```python
from build123d import *

# Parameters (mm, degrees)
SKETCH1_W           = 25.4
SKETCH1_H           = 25.4
BOSS_EXTRUDE1_DEPTH = 482.6
SKETCH2_R           = 6.35
BOSS_EXTRUDE2_DEPTH = 6.35
SKETCH3_R           = 6.35
BOSS_EXTRUDE3_DEPTH = 6.35
SKETCH4_W           = 25.4
SKETCH4_H           = 482.6
BOSS_EXTRUDE4_DEPTH = 18.288


with BuildPart() as part:
    # Sketch1 → Boss-Extrude1 (new body)
    with BuildSketch(Plane(origin=(0, 0, 0), x_dir=(1, 0, 0), z_dir=(0, 1, 0))):
        with Locations((12.7, 12.7)):
            Rectangle(SKETCH1_W, SKETCH1_H)
    extrude(amount=BOSS_EXTRUDE1_DEPTH)

    # Sketch2 → Boss-Extrude2 (add)
    with BuildSketch(Plane(origin=(25.4, 0, 0), x_dir=(0, 0, -1), z_dir=(1, 0, 0))):
        with Locations(Location((12.7, 469.9, 0), (0, 0, 180))):
            Circle(SKETCH2_R)
    extrude(amount=BOSS_EXTRUDE2_DEPTH)

    # Sketch3 → Boss-Extrude3 (add)
    with BuildSketch(Plane(origin=(25.4, 0, 0), x_dir=(0, 0, -1), z_dir=(1, 0, 0))):
        with Locations(Location((12.7, 12.7, 0), (0, 0, 180))):
            Circle(SKETCH3_R)
    extrude(amount=BOSS_EXTRUDE3_DEPTH)

    # Sketch4 → Boss-Extrude4 (add)
    with BuildSketch(Plane(origin=(0, 0, -25.4), x_dir=(-1, 0, 0), z_dir=(0, 0, -1))):
        with Locations((-12.7, 241.3)):
            Rectangle(SKETCH4_W, SKETCH4_H)
    extrude(amount=BOSS_EXTRUDE4_DEPTH)


solid = part.part
```
Check sheet for the modelled part. Datum: model origin and axes. Units: mm. Give positions to 0.01 mm unless a question says otherwise; leave off trailing zeros. Write each loop counter-clockwise with the first axis right and the second up, starting at its lowest first coordinate (ties: lowest second). Pieces come first, ordered by that corner, then holes. Notation, with made-up numbers: (81, 40) - (121, 40) arc R24 cw to (121, 76) - close; hole circle Ø1 at (63.5, -38). An arc over 180 degrees is marked (long way). Answer as a JSON object with one key per item and string values. Group by question number.
1) Depth check by flat-ended pin: P1, Ø8, axis at y = 247, z = -17, coming from the +X side; P2, Ø1.5, axis at x = 15.5, z = -35.5, coming from the -Y side. Enter the tip coordinate at first touch or a pass-through.
2) Sectioned sample at B-B (y = 12.7). Record the cut outline in (x, z), then the cut area to 3 significant figures.
3) Release check for a two-part mould opening along Y. For faces 1 (the face through (13, 0, -22)), 2 (the face through (13, 245, -43.688)), 3 (the face through (28.5, 463.6, -13.5)), 4 (the face through (28.53, 18.9, -14.08)) record: pulls with the +Y half, pulls with the -Y half, needs draft (parallel to the pull), parting line crosses it, or undercut.
4) Thickness scan on probe 1 along Y at (x, z) = (27.5, -13); probe 2 along X at (y, z) = (85, -36.5); probe 3 along Y at (x, z) = (30, -17.5). Record the ranges inside material, lowest first. Write a range as from..to.
5) Sectioned sample at C-C (z = -37). Record the cut outline in (x, y).
6) Sectioned sample at A-A (z = -12.7). Record the cut outline in (x, y).
Geometry results:
{
 "1": {"P1": "stops at x = 25.4", "P2": "stops at y = 0"},
 "2": {"outline": "(0, -43.69) - (25.4, -43.69) - (25.4, -19.05) - (31.75, -19.05) - (31.75, -6.35) - (25.4, -6.35) - (25.4, 0) - (0, 0) - close", "area": "1,190 mm^2"},
 "3": {"face 1": "pulls with the -Y half", "face 2": "needs draft", "face 3": "undercut", "face 4": "undercut"},
 "4": {"probe 1": "y = 6.36..19.04, 463.56..476.24", "probe 2": "x = 0..25.4", "probe 3": "y = 8.54..16.86, 465.74..474.06"},
 "5": {"outline": "(0, 0) - (25.4, 0) - (25.4, 482.6) - (0, 482.6) - close"},
 "6": {"outline": "(0, 0) - (25.4, 0) - (25.4, 6.35) - (31.75, 6.35) - (31.75, 19.05) - (25.4, 19.05) - (25.4, 463.55) - (31.75, 463.55) - (31.75, 476.25) - (25.4, 476.25) - (25.4, 482.6) - (0, 482.6) - close"}
}
